Could you check a few things on this model? Use its own coordinates, in mm. Face numbers are marked on the shaded views. A direction names the side the tool comes from. Give positions to 0.01 mm unless a question says otherwise; leave off trailing zeros. Order: outer loops, then holes, each group sorted by start corner. A loop starts at its lowest first (then second) coordinate and runs counter-clockwise, first axis right, second up. Notation, with made-up numbers: (87, -22) -> (118, -22) arc R21 ccw to (118, 2) -> close; hole circle Ø2 at (13.5, -27). An arc over 180 degrees is marked (long way). Use one line per item in the form item = value. Start each with the question number.
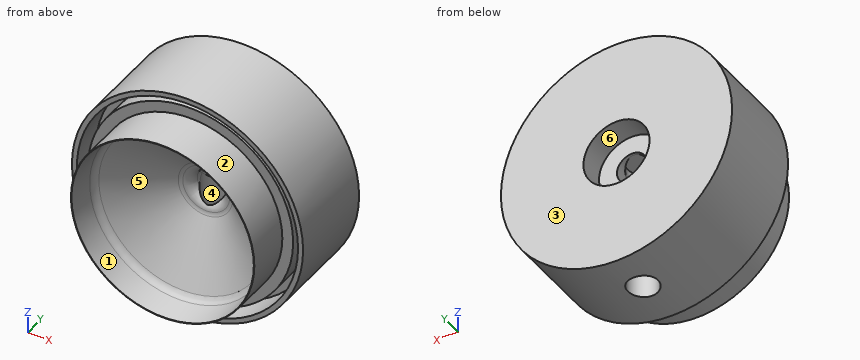
Autodesk Inventor part; units mm, degrees
ref_plane "YZ Plane" through (0, 0, 0) normal (1, 0, 0) x (0, 1, 0)
ref_plane "XZ Plane" through (0, 0, 0) normal (0, 1, 0) x (-1, 0, 0)
ref_plane "XY Plane" through (0, 0, 0) normal (0, 0, 1) x (1, 0, 0)
sketch "Sketch1" plane through (0, 0, 0) normal (0, 0, 1) x (1, 0, 0)
  line L0 (3, 12) -> (23, 12)
  line L1 (23, 12) -> (23, 0)
  line L2 (3, 2) -> (3, 12)
  line L3 (0, 19.5472) -> (0, -22.4151)
  line L4 (23, 0) -> (22, 0) construction
  line L5 (22, 0) -> (22, -6)
  line L6 (22, -6) -> (23, -6)
  line L7 (23, -6) -> (23, 0)
  line L8 (20.4, 0) -> (17.25, 0) construction
  line L9 (17.25, 0) -> (17.25, -5) construction
  line L10 (17.25, -5) -> (20.4, -5) construction
  line L11 (20.4, -5) -> (20.4, 0)
  arc A0 (3, 2) -> (4.6637, 0.0285) centre (5, 2) ccw
  line L12 (22, 0) -> (20.4, 0)
  line L13 (17.25, 0) -> (5, 0)
  line L14 (-20.0393, 0) -> (22, 0) construction
  line L15 (23, 0) -> (24.5476, 0) construction
  line L16 (18.25, 0) -> (18.25, -5) construction
  line L17 (20.4, -5) -> (18.25, -5)
  line L18 (18.25, -5) -> (18.25, -14)
  line L19 (18.25, -14) -> (18.15, -14)
  line L20 (18.15, -14) -> (17.25, -5) construction
  line L21 (18.25, -8) -> (17.55, -8) construction
  line L22 (5.4025, -0.2566) -> (16.7316, -7.4783)
  line L23 (17.6466, -8.9658) -> (18.15, -14)
  arc A1 (17.6466, -8.9658) -> (16.7316, -7.4783) centre (15.6565, -9.1648) ccw
  arc A2 (5.4025, -0.2566) -> (4.6637, 0.0285) centre (4.3274, -1.943) ccw
  point P0 (0, 0)
  point P1 (17.25, 0)
  point P2 (17.25, -5)
  point P3 (5, 0)
  point P4 (17.9, -8)
  dimension "d0" = 6
  dimension "d2" = 1
  dimension "d5" = 5
  dimension "d6" = 1.6
  dimension "d7" = 44
  dimension "d11" = 2
  dimension "d12" = 12
  dimension "d14" = 6
  dimension "d23" = 36.5
  dimension "d24" = 1
  dimension "d25" = 0.1
  dimension "d26" = 9
  dimension "d37" = 3
  dimension "d38" = 2
  dimension "d39" = 2
revolve "Revolution1" add sketch "Sketch1" angle 360 about axis through (0, 19.5472, 0) along (0, -1, 0)
sketch "Sketch2" plane through (0, 0, 0) normal (0, 0, 1) x (1, 0, 0)
  line L0 (-3, 12) -> (3, 12)
  line L1 (0, 12) -> (0, 0) construction
  line L2 (-3, 2) -> (3, 2) construction
  circle A0 centre (0, 3.5) radius 3
  line L3 (-20.4, 0) -> (20.4, 0)
  point P0 (2.5981, 2)
  point P1 (-2.5981, 2)
  dimension "d16" = 6
  dimension "d40" = 3.5
extrude "Extrusion1" cut sketch "Sketch2" along normal blind 3 and the other way blind 33
sketch "Sketch3" plane through (0, 12, 0) normal (0, 1, 0) x (1, 0, 0)
  circle A0 centre (0, 0) radius 6.575
  circle A1 centre (0, 0) radius 3 construction
  dimension "d27" = 13.15
extrude "Extrusion2" cut sketch "Sketch3" against normal blind 5
equation "\"d0\" = t_D"
equation "\"d2\" = w_th"
equation "\"d5\" = b_rim_h"
equation "\"d6\" = lv_th"
equation "\"d7\" = b_OD"
equation "\"d11\" = fillet_D"
equation "\"d12\" = top_th_f"
equation "\"d14\" = w_l"
equation "\"d23\" = b_ID"
equation "\"d24\" = w_th"
equation "\"d25\" = tol"
equation "\"d26\" = 1.5 * w_l"
equation "\"d38\" = fillet_D"
equation "\"d39\" = fillet_D"
equation "\"d16\" = t_D"
equation "\"d40\" = 0.5 * w_th + 0.5 * t_D"
equation "\"d18\" = 0.5 * t_D"
equation "\"d19\" = 0.75 * b_OD"
equation "\"d27\" = cn_D"
equation "\"d30\" = cn_h"
equation "\"tol\" = 0.1"
equation "\"fillet_D\" = 2"
equation "\"w_th\" = 1"
equation "\"w_l\" = 6"
equation "\"t_D\" = 6"
equation "\"t_D_f\" = t_D + w_th"
equation "\"top_th_f\" = t_D_f + cn_h"
equation "\"cn_h\" = 5"
equation "\"lv_th\" = 1.6"
equation "\"d3\" = w_l"
equation "\"d8\" = top_th_f"
equation "\"b_ID\" = 36.5"
equation "\"b_OD\" = 44"
equation "\"b_rim_h\" = 5"
equation "\"top_th\" = t_D + w_th"
equation "\"lv_OD\" = 26"
equation "\"sv_OD\" = 13"
equation "\"sv_th\" = 1.5"
equation "\"b_th\" = 1.5"
equation "\"h_s\" = 2.25"
equation "\"h_D\" = 0.75"
equation "\"v_h_D\" = 7.5"
equation "\"v_h_off\" = 0.5 * cn_D + 0.5 * v_h_D"
properties part number "bottle"
(1) We'd pull the mould along Y, two halves only. Please class the marked faces 1, 2, 3 and 4: pulls with the +Y half, pulls with the -Y half, needs draft (parallel to the pull), parting line crosses it, or undercut.
(2) Imagine slicing it at C-C (y = -3). Write out the boundary of the cut face in (x, z), plus the area to 3 significant figures.
(3) Imagine slicing it at A-A (x = 19). Write out the boundary of the cut face in (y, z), plus the area to 3 significant figures.
(4) Please list where these lines run through material, in increasing order: probe 1 along Z at (x, y) = (4.5, -5.5); probe 2 along X at (y, z) = (-1.5, 18.5); probe 3 along X at (y, z) = (-2, 4.5).
(5) Which directions (+Z, -Z, +X, -X, +Y, -Y) give clear straight access to the entire face, cutting with the end or side of a thin tool? Please do the marked faces 5 and 6.
(6) I'm going to push flat-ended pins straight in: pin 1 Ø8 at (x, y) = (-9.5, -4) entering from +Z; pin 2 Ø2 at (y, z) = (5, -15) entering from -X; pin 3 Ø2 at (x, y) = (-0.5, 6) entering from +Z; pin 4 Ø3 at (x, y) = (0.5, 5) entering from -Z. Where does each tip first touch, or does it pass through?
(7) Imagine slicing it at D-D (z = 19). Write out the boundary of the cut face in (x, y), plus the area to 3 significant figures.
(8) Imagine slicing it at B-B (y = 10). Write out the boundary of the cut face in (x, z) (3 decimals), plus the area to 3 significant figures.
Calculated:
q1.face_1 = pulls with the -Y half
q1.face_2 = needs draft
q1.face_3 = pulls with the +Y half
q1.face_4 = undercut
q2.outline = circle Ø46 at (0, 0); circle Ø40.8 at (0, 0); hole circle Ø44 at (0, 0); hole circle Ø19.41 at (0, 0)
q2.area = 1,150 mm2
q3.outline = (-6, -12.96) -> (12, -12.96) -> (12, 12.96) -> (-6, 12.96) -> (-6, 11.09) -> (0, 11.09) -> (0, 7.43) -> (-5, 7.43) -> (-5, -7.43) -> (0, -7.43) -> (0, -11.09) -> (-6, -11.09) -> close
q3.area = 408 mm2
q4.probe_1 = -22.56 to -21.53, -17.69 to -12.86, 12.86 to 17.69, 21.53 to 22.56
q4.probe_2 = -13.67 to -11.91, -8.6 to 8.6, 11.91 to 13.67
q4.probe_3 = -22.56 to -21.53, -19.9 to -6.78, 6.78 to 19.9, 21.53 to 22.56
q5.face_5 = -Y
q5.face_6 = +Y
q6.pin_1 = 22.33
q6.pin_2 = -18.25
q6.pin_3 = 23
q6.pin_4 = -23
q7.outline = (-12.96, -6) -> (-11.09, -6) -> (-11.09, 0) -> (-7.43, 0) -> (-7.43, -5) -> (7.43, -5) -> (7.43, 0) -> (11.09, 0) -> (11.09, -6) -> (12.96, -6) -> (12.96, 12) -> (-12.96, 12) -> close
q7.area = 408 mm2
q8.outline = circle Ø46 at (0, 0); hole circle Ø13.15 at (0, 0)
q8.area = 1,530 mm2
